Study the drawing (mm; zero at the part's minimum x, y, z) and answer. A direction names the side the tool comes from. Round coordinates to 2 decimals unless told otherwise and drop trailing zeros. Write each loop counter-clockwise with the first axis right and the second up, starting at its lowest first coordinate (ties: lowest second). Pieces come first, ordered by that corner, then holes. Notation, with made-up numbers: M 19,49.5 L 71,49.5 A30 cw 71,81.5 Z; hole C -4.75,50.5 d9. An arc over 180 degrees is marked long. Put each result on its own line as item: value. Start each with the question number.
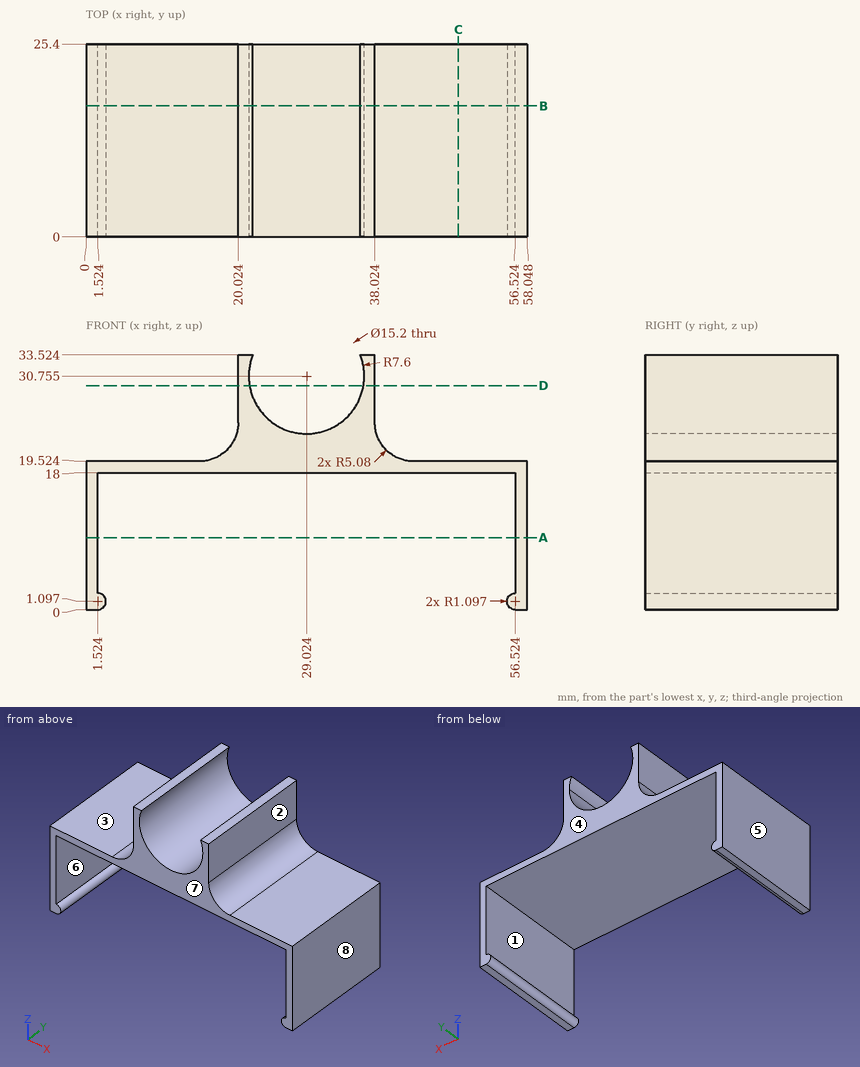
Item 1: Section A-A (z = 9.5) is taken. Give the vertices of the cut face in (x, y).
Item 2: Section D-D (z = 29.5) is taken. Give the vertices of the cut face in (x, y).
Item 3: Determine the mould class of the marked faces 6, 7 and 8 for opening direction X: released by +X, released by -X, zero draft, split by the parting line, or undercut.
Item 4: Flat-ended cylindrical pins translate along their axes: pin 1 (7.5 mm diameter, centred on x = 52, y = 12.5, fed in from +Z); pin 2 (7 mm diameter, centred on y = 17, z = 28.5, fed in from -X); pin 3 (4.5 mm diameter, centred on y = 18, z = 10.5, fed in from -X); pin 4 (5 mm diameter, centred on y = 22.5, z = 24, fed in from +X). Find the tip coordinate at first contact, or state that the pin passes through.
Item 5: Which of the six approach directions +Z, -Z, +X, -X, +Y, -Y give full straight-line access (tool end or side, diameter ignored) to the marked faces 1, 2, 3, 4 and 5?
Item 6: Consider line 1 along X through (y, z) = (14, 10.5); line 2 along X through (y, z) = (15.25, 28) (1 decimal); line 3 along Z through (x, y) = (12, 4). Determine where each line is inside the solid, lowest interval first. Write a range as [from, to].
Item 7: Section C-C (x = 49) is taken. Give the vertices of the cut face in (y, z).
Item 8: Section B-B (y = 17.25) is taken. Give the vertices of the cut face in (x, z) (1 decimal).
Output values:
1. outline: M 0,0 L 1.52,0 L 1.52,25.4 L 0,25.4 Z; M 56.52,0 L 58.05,0 L 58.05,25.4 L 56.52,25.4 Z
2. outline: M 20.02,0 L 21.53,0 L 21.53,25.4 L 20.02,25.4 Z; M 36.52,0 L 38.02,0 L 38.02,25.4 L 36.52,25.4 Z
3. face 6: undercut
3. face 7: zero draft
3. face 8: released by +X
4. pin 1: stops at z = 19.52
4. pin 2: stops at x = 20.02
4. pin 3: stops at x = 0
4. pin 4: stops at x = 39.08
5. face 1: +Y, -Y
5. face 2: +Z, +X, +Y, -Y
5. face 3: +Z, -X, +Y, -Y
5. face 4: +Z, -Z, +X, -X, +Y
5. face 5: +Z, -Z, -X, +Y, -Y
6. line 1: x = [0, 1.52], [56.52, 58.05]
6. line 2: x = [20, 21.9], [36.1, 38]
6. line 3: z = [18, 19.52]
7. outline: M 0,18 L 25.4,18 L 25.4,19.52 L 0,19.52 Z
8. outline: M 0,0 L 1.5,0 A1.1 ccw 1.5,2.2 L 1.5,18 L 56.5,18 L 56.5,2.2 A1.1 ccw 56.5,0 L 58,0 L 58,19.5 L 43.1,19.5 A5.1 cw 38,24.6 L 38,33.5 L 36.1,33.5 A7.6 cw long 21.9,33.5 L 20,33.5 L 20,24.6 A5.1 cw 14.9,19.5 L 0,19.5 Z
